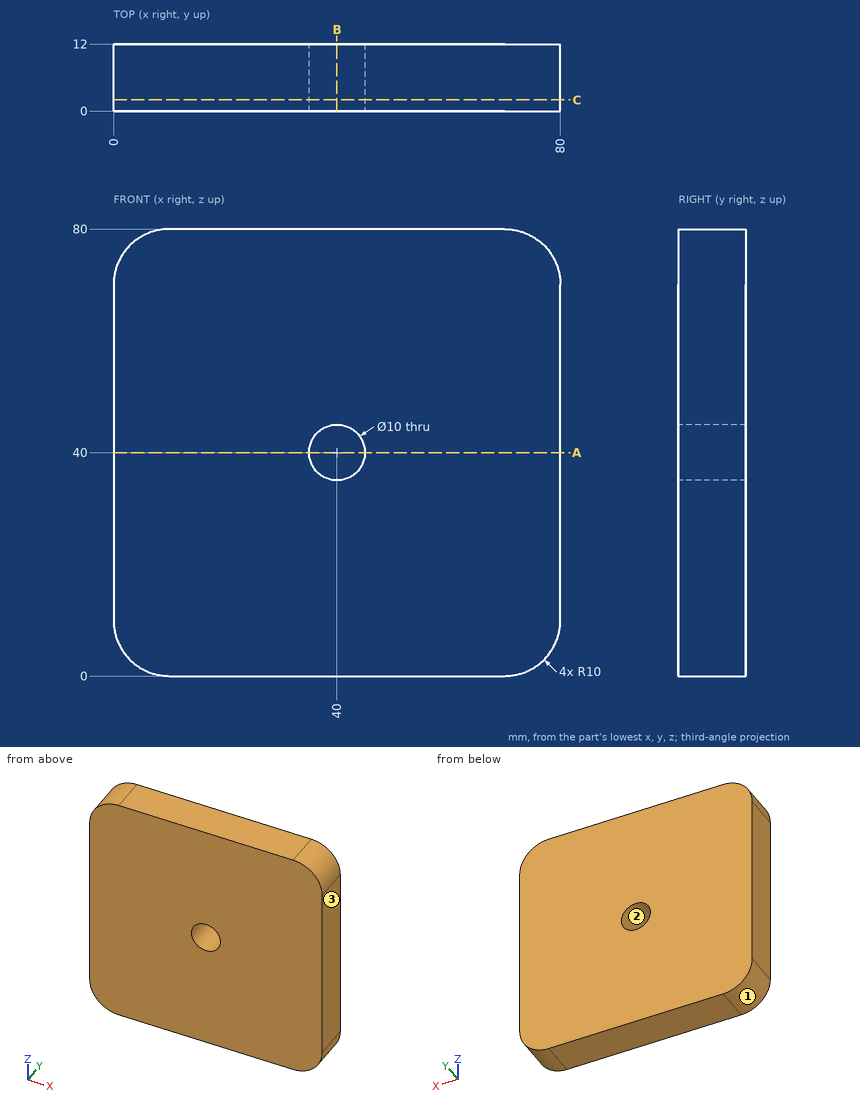
Here's the drawing with two shaded views (mm, measured from the low corner). I have some questions. Coordinates: 2 decimals unless noted, no trailing zeros. Loops run counter-clockwise (first coordinate to the right, second up) from the corner with the lowest first, then second, coordinate; pieces in that order, holes last.
Item 1: If we mould it in two halves opening along X, with no side actions, what happens to the marked faces 1, 2 and 3? For each: released by +X, released by -X, zero draft, split by the parting line, or undercut.
Answers below:
face 1: released by -X
face 2: undercut
face 3: released by +X
Item 2: Please list where these lines run through material, in increasing order: L1, parallel to Z at x = 40, y = 3.5; L2, parallel to Z at x = 38.5, y = 3.5; L3, parallel to Z at x = 3.5, y = 4.25.
Answers below:
L1: z = 0 to 35, 45 to 80
L2: z = 0 to 35.23, 44.77 to 80
L3: z = 2.4 to 77.6
Item 3: I'm going to push a flat-ended pin straight in: pin 1 (1.5 mm diameter, centred on x = 57.5, z = 64, fed in from -Y). Where does the tip first touch, or does it pass through?
Answers below:
pin 1: stops at y = 0
Item 4: Suppose I cut it at B-B (x = 40). Please give me the cut outline in (y, z), then the cut area to 3 significant figures.
Answers below:
outline: (0, 0) - (12, 0) - (12, 35) - (0, 35) - close; (0, 45) - (12, 45) - (12, 80) - (0, 80) - close
area: 840 mm2
Item 5: Suppose I cut it at C-C (y = 2). Please give me the cut outline in (x, z).
Answers below:
outline: (0, 10) arc R10 ccw to (10, 0) - (70, 0) arc R10 ccw to (80, 10) - (80, 70) arc R10 ccw to (70, 80) - (10, 80) arc R10 ccw to (0, 70) - close; hole circle Ø10 at (40, 40)
Item 6: Suppose I cut it at A-A (z = 40). Please give me the cut outline in (x, y), then the cut area to 3 significant figures.
Answers below:
outline: (0, 0) - (35, 0) - (35, 12) - (0, 12) - close; (45, 0) - (80, 0) - (80, 12) - (45, 12) - close
area: 840 mm2
